The listing builds one solid part. Answer for the finished solid, in the listing's coordinates (mm). A direction names the side the tool comes from. Give positions to 0.01 mm unless a question says otherwise; leave off trailing zeros. Order: outer loops, then holes, each group sorted by start corner. A loop starts at its lowest first (then second) coordinate and runs counter-clockwise, first axis right, second up. Notation, with made-up numbers: (79.25, 79.5) - (133.25, 79.5) arc R26 ccw to (133.25, 109.5) - close; hole circle Ø5 at (77, -19.75). An arc over 180 degrees is marked (long way). Answer as a JSON object with one key per item and string values. Group by question number.
Q1. A cutting plane is placed at C-C, the plane x = 0. Give the vertices of the cut face in (y, z).
Q2. A cutting plane is placed at A-A, the plane z = 0. Give the vertices of the cut face in (x, y), and give its area (3 significant figures).
Q3. The mould has two halves that part along Z. Classify faces 1 (the face through (0, -19, 0)), 2 (the face through (-1.4, -26, 0)), 3 (the face through (3.233, -14.297, -1.341)): released by +Z, released by -Z, zero draft, split by the parting line, or undercut.
Q4. Given pin 1 (1.9 mm diameter, centred on y = -24.5, z = 0.5, fed in from +X); pin 2 (3 mm diameter, centred on x = 2, y = -6.5, fed in from +Z); pin 3 (1.4 mm diameter, centred on x = 0, z = 1, fed in from -Y); pin 4 (4 mm diameter, centred on x = 1.5, y = -24, fed in from -Z), each flat-ended and moving along its own axis, determine where each tip first touches the part or whether it passes through.
Q5. For faces 4 (the face through (0, -22.167, 0)), 5 (the face through (2, -29, 0)), 6 (the face through (0, -9, -2)), determine the directions among +Z, -Z, +X, -X, +Y, -Y from which every point of the face is accessible in a straight line to the end or side of a thin tool.
Q6. Consider line 1 (Z direction, x = 0, y = -9.5); line 2 (Y direction, x = 1, z = 2); line 3 (Z direction, x = -1.75, y = -8.75). Determine where each line is inside the solid, lowest interval first.
Q7. A cutting plane is placed at B-B, the plane y = -22.5. Give the vertices of the cut face in (x, z).
Q8. A cutting plane is placed at D-D, the plane y = -10.5. Give the vertices of the cut face in (x, z), and give its area (3 significant figures).
from build123d import *

# Parameters (mm, degrees)
F1_R     = 3.5
F2_DEPTH = 29
F0_R     = 2
F3_DEPTH = 19
F4_W     = 2.8
F4_H     = 7.9
F5_DEPTH = 12.5


with BuildPart() as f2:
    # F1 (on Front) → F2 (new body)
    with BuildSketch(Plane.XZ):
        Circle(F1_R)
    extrude(amount=F2_DEPTH)

    # F0 (on Front) → F3 (cut)
    with BuildSketch(Plane.XZ):
        Circle(F0_R)
    extrude(amount=F3_DEPTH, mode=Mode.SUBTRACT)

    # F4 (on Top) → F5 (cut, symmetric)
    with BuildSketch(Plane.XY):
        with Locations((0, -26.117409)):
            Rectangle(F4_W, F4_H)
    extrude(amount=F5_DEPTH, both=True, mode=Mode.SUBTRACT)


solid = f2.part
Reply:
{
 "1": {"outline": "(-22.17, -3.5) - (0, -3.5) - (0, -2) - (-19, -2) - (-19, 2) - (0, 2) - (0, 3.5) - (-22.17, 3.5) - close"},
 "2": {"outline": "(-3.5, -29) - (-1.4, -29) - (-1.4, -22.17) - (1.4, -22.17) - (1.4, -29) - (3.5, -29) - (3.5, 0) - (2, 0) - (2, -19) - (-2, -19) - (-2, 0) - (-3.5, 0) - close", "area": "108 mm^2"},
 "3": {"face 1": "undercut", "face 2": "zero draft", "face 3": "split by the parting line"},
 "4": {"pin 1": "stops at x = 3.5", "pin 2": "stops at z = 3.46", "pin 3": "stops at y = -22.17", "pin 4": "stops at z = -3.43"},
 "5": {"face 4": "+Z, -Z, -Y", "face 5": "+Z, -Z, +X, -X, -Y", "face 6": "+Y"},
 "6": {"line 1": "z = -3.5 to -2, 2 to 3.5", "line 2": "y = -22.17 to 0", "line 3": "z = -3.03 to -0.97, 0.97 to 3.03"},
 "7": {"outline": "(-1.4, -3.21) - (-1.4, 3.21) arc R3.5 ccw to start; (1.4, -3.21) arc R3.5 ccw to (1.4, 3.21) - close"},
 "8": {"outline": "circle Ø7 at (0, 0); hole circle Ø4 at (0, 0)", "area": "25.9 mm^2"}
}
